Work out the finished part from the listing and answer in its coordinate system (mm). A direction names the side the tool comes from. Give positions to 0.01 mm unless a question says otherwise; leave off trailing zeros. Loops run counter-clockwise (first coordinate to the right, second up) from the corner with the lowest first, then second, coordinate; pieces in that order, holes last.
from build123d import *

# Parameters (mm, degrees)
F0_W     = 60
F0_H     = 20
F0_R     = 0.75
F1_DEPTH = 3


with BuildPart() as f1:
    # F0 (on Top) → F1 (new body)
    with BuildSketch(Plane.XY):
        Rectangle(F0_W, F0_H)
        with BuildLine():
            ThreePointArc((-23.55, -5), (-24.83033, -5.53033), (-24.3, -4.25))
            ThreePointArc((-24.3, -4.25), (-23.76967, -4.46967), (-23.55, -5))
        make_face(mode=Mode.SUBTRACT)
        with Locations((24.3, -5)):
            Circle(F0_R, mode=Mode.SUBTRACT)
        with Locations((-17.5, 0)):
            Circle(F0_R, mode=Mode.SUBTRACT)
        with BuildLine():
            ThreePointArc((-23.55, 5), (-23.76967, 4.46967), (-24.3, 4.25))
            ThreePointArc((-24.3, 4.25), (-24.83033, 5.53033), (-23.55, 5))
        make_face(mode=Mode.SUBTRACT)
        with BuildLine():
            ThreePointArc((-14.1, 5.5), (-13.807107, 6.207107), (-13.1, 6.5))
            Line((-13.1, 6.5), (13.1, 6.5))
            ThreePointArc((13.1, 6.5), (13.807107, 6.207107), (14.1, 5.5))
            Line((14.1, 5.5), (14.1, -5.5))
            ThreePointArc((14.1, -5.5), (13.807107, -6.207107), (13.1, -6.5))
            Line((13.1, -6.5), (-13.1, -6.5))
            ThreePointArc((-13.1, -6.5), (-13.807107, -6.207107), (-14.1, -5.5))
            Line((-14.1, -5.5), (-14.1, 5.5))
        make_face(mode=Mode.SUBTRACT)
        with Locations((17.5, 0)):
            Circle(F0_R, mode=Mode.SUBTRACT)
        with Locations((24.3, 5)):
            Circle(F0_R, mode=Mode.SUBTRACT)
    extrude(amount=F1_DEPTH)


solid = f1.part
Item 1: Find section A-A, the plane y = 0. Write down the section's boundary in (x, z).
Item 2: Consider line 1 (Y direction, x = 24.3, z = 1.6); line 2 (Y direction, x = 9, z = 2.3); line 3 (Y direction, x = -17.5, z = 1.5). Determine where each line is inside the solid, lowest interval first.
Item 3: Find section C-C, the plane z = 2.15. Write down the section's boundary in (x, y).
Item 4: Find section D-D, the plane y = -2.5. Write down the section's boundary in (x, z).
Item 5: A flat-ended cylindrical pin translates along its axis: pin 1 Ø2 at (x, y) = (24.3, -5) entering from +Z. Find the tip coordinate at first contact, or state that the pin passes through.
Item 6: Find section B-B, the plane x = 17.5. Write down the section's boundary in (y, z), plus the area to 3 significant figures.
Item 7: Determine the mould class of faces 1 (the face through (0, 7, 3)), 2 (the face through (13.799, 6.215, 1.479)), 3 (the face through (30, 0, 1)) for opening direction X: released by +X, released by -X, zero draft, split by the parting line, or undercut.
Item 8: For faces 4 (the face through (0, 10, 1)), 5 (the face through (0, -6.5, 1)), determine the directions among +Z, -Z, +X, -X, +Y, -Y from which every point of the face is accessible in a straight line to the end or side of a thin tool.
Ans:
1. outline: (-30, 0) - (-18.25, 0) - (-18.25, 3) - (-30, 3) - close; (-16.75, 0) - (-14.1, 0) - (-14.1, 3) - (-16.75, 3) - close; (14.1, 0) - (16.75, 0) - (16.75, 3) - (14.1, 3) - close; (18.25, 0) - (30, 0) - (30, 3) - (18.25, 3) - close
2. line 1: y = -10 to -5.75, -4.25 to 4.25, 5.75 to 10
2. line 2: y = -10 to -6.5, 6.5 to 10
2. line 3: y = -10 to -0.75, 0.75 to 10
3. outline: (-30, -10) - (30, -10) - (30, 10) - (-30, 10) - close; hole circle Ø1.5 at (-24.3, -5); hole circle Ø1.5 at (-24.3, 5); hole circle Ø1.5 at (-17.5, 0); hole (-14.1, -5.5) arc R1 ccw to (-13.1, -6.5) - (13.1, -6.5) arc R1 ccw to (14.1, -5.5) - (14.1, 5.5) arc R1 ccw to (13.1, 6.5) - (-13.1, 6.5) arc R1 ccw to (-14.1, 5.5) - close; hole circle Ø1.5 at (17.5, 0); hole circle Ø1.5 at (24.3, -5); hole circle Ø1.5 at (24.3, 5)
4. outline: (-30, 0) - (-14.1, 0) - (-14.1, 3) - (-30, 3) - close; (14.1, 0) - (30, 0) - (30, 3) - (14.1, 3) - close
5. pin 1: stops at z = 3
6. outline: (-10, 0) - (-0.75, 0) - (-0.75, 3) - (-10, 3) - close; (0.75, 0) - (10, 0) - (10, 3) - (0.75, 3) - close
6. area: 55.5 mm2
7. face 1: zero draft
7. face 2: undercut
7. face 3: released by +X
8. face 4: +Z, -Z, +X, -X, +Y
8. face 5: +Z, -Z
